For this review, take the finished solid that the model builds, in its own axes (mm). Face numbers are marked on the shaded views. A direction names the side the tool comes from. Round coordinates to 2 decimals unless told otherwise and drop trailing zeros. Write each loop counter-clockwise with the first axis right and the second up, starting at its lowest first coordinate (ties: lowest second). Pieces come first, ordered by that corner, then holes. Notation, with made-up numbers: (20.25, -39) -> (71.25, -39) arc R11 ccw to (71.25, -30) -> close; hole circle Ø4 at (77, 63). An arc over 180 degrees is marked (long way). Write each question's results on one line, items separated by ' | '. Start each with the question number.
Item 1: Add section A-A (x = -21.5). State the section outline as (y, z) points.
Item 2: Tool access review of the marked faces 1, 2 and 3: name each direction out of +Z, -Z, +X, -X, +Y, -Y from which nothing blocks a thin tool from reaching the whole face with its end or side.
Item 3: Clearance check with flat-ended pins moving along their axes: pin 1 (3 mm diameter, centred on x = -16.5, z = -11.5, fed in from -Y); pin 2 (12 mm diameter, centred on y = 125, z = -26, fed in from +X). State where each tip first meets the part, or that it passes through.
Item 4: Add section C-C (x = -3). State the section outline as (y, z) points, plus the area to 3 significant figures.
Item 5: To check wall thickness, follow line 1 along Y through (x, z) = (-8.5, -36); line 2 along Y through (x, z) = (-12, -21.5); line 3 along Z through (x, y) = (-29, 125) (3 decimals). State the ranges of each line that lie inside material, in increasing order.
Item 6: Add section B-B (z = -7.5). State the section outline as (x, y) points, plus the area to 3 significant figures.
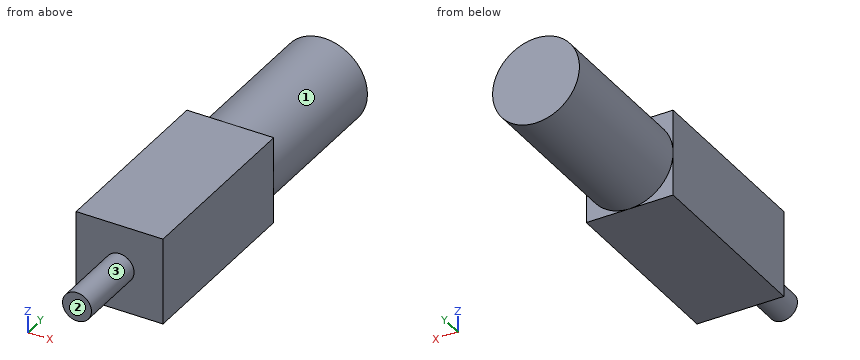
Autodesk Inventor part; units mm, degrees
ref_plane "YZ Plane" through (0, 0, 0) normal (1, 0, 0) x (0, 1, 0)
ref_plane "XZ Plane" through (0, 0, 0) normal (0, 1, 0) x (-1, 0, 0)
ref_plane "XY Plane" through (0, 0, 0) normal (0, 0, 1) x (1, 0, 0)
sketch "Sketch1" plane through (0, 0, 0) normal (0, 1, 0) x (-1, 0, 0)
  line L0 (0, 0) -> (38.1, 0)
  line L1 (38.1, 0) -> (38.1, -38.1)
  line L2 (38.1, -38.1) -> (0, -38.1)
  line L3 (0, -38.1) -> (0, 0)
  dimension "d0" = 38.1
  dimension "d1" = 38.1
extrude "Extrusion1" add sketch "Sketch1" along normal blind 82.55
sketch "Sketch2" plane through (0, 82.55, 0) normal (0, 1, 0) x (1, 0, 0)
  circle A0 centre (-19.05, 19.05) radius 19.05
  line L0 (-38.1, 0) -> (-38.1, 38.1)
  line L1 (-38.1, 38.1) -> (0, 38.1)
  point P0 (0, 0)
  dimension "d4" = 38.1
  dimension "d5" = 19.05
  dimension "d6" = 19.05
extrude "Extrusion2" add sketch "Sketch2" along normal blind 69.85 contours A0
sketch "Sketch3" plane through (0, 0, 0) normal (0, -1, 0) x (1, 0, 0)
  circle A0 centre (-19.05, -19.05) radius 6.35
  line L0 (0, 0) -> (-38.1, 0)
  line L1 (-38.1, 0) -> (-38.1, -38.1)
  dimension "d9" = 12.7
  dimension "d10" = 19.05
  dimension "d11" = 19.05
extrude "Extrusion3" add sketch "Sketch3" along normal blind 31.75
properties part number "articulation motor 300 to 1"
Responses:
1) outline: (-31.75, -24.91) -> (0, -24.91) -> (0, -38.1) -> (82.55, -38.1) -> (82.55, -37.94) -> (152.4, -37.94) -> (152.4, -0.16) -> (82.55, -0.16) -> (82.55, 0) -> (0, 0) -> (0, -13.19) -> (-31.75, -13.19) -> close
2) face 1: +Y | face 2: +Z, -Z, +X, -X, -Y | face 3: -Y
3) pin 1: stops at y = 0 | pin 2: stops at x = -0.02
4) outline: (0, -38.1) -> (82.55, -38.1) -> (82.55, -29.31) -> (152.4, -29.31) -> (152.4, -8.79) -> (82.55, -8.79) -> (82.55, 0) -> (0, 0) -> close | area: 4,580 mm^2
5) line 1: y = 0 to 82.55 | line 2: y = 0 to 152.4 | line 3: z = -35.295 to -2.805
6) outline: (-38.1, 0) -> (0, 0) -> (0, 82.55) -> (-3.9, 82.55) -> (-3.9, 152.4) -> (-34.2, 152.4) -> (-34.2, 82.55) -> (-38.1, 82.55) -> close | area: 5,260 mm^2
